Build history of the part. All positions in model axes, mm. Round coordinates to 2 decimals unless told otherwise and drop trailing zeros. Loops run counter-clockwise (first coordinate to the right, second up) from the corner with the lowest first, then second, coordinate; pieces in that order, holes last. Notation, with made-up numbers: (20.25, 50.25) - (52.25, 50.25) arc R7 cw to (52.25, 55.25) - close; hole circle Ø7 at (23, 40.5). An arc over 180 degrees is marked (long way). Use one line per item in the form item = value. Start each with the question number.
Q1. Drill centre lines: line 1 (X direction, y = 1.95, z = -15); line 2 (Z direction, x = 1.5, y = 0.5); line 3 (X direction, y = 2.05, z = 0). Where is each one in solid material? Low to high.
Q2. Pin check, flat tip, straight feed: pin 1 (5 mm diameter, centred on x = 0, z = 30, fed in from +Y). Stop position of the tip, or through.
Q3. Saw through at C-C (x = 26). Give the cut face in (y, z), then the cut area to 3 significant figures.
Q4. Saw through at A-A (y = 1). Give the cut face in (x, z), then the cut area to 3 significant figures.
Q5. Saw through at D-D (z = -15). Give the cut face in (x, y), then the cut area to 3 significant figures.
Q6. Saw through at B-B (z = 30). Give the cut face in (x, y), then the cut area to 3 significant figures.
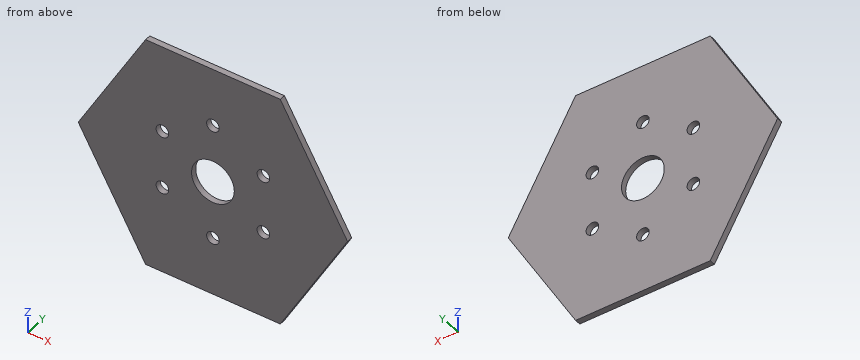
```python
from build123d import *

# Parameters (mm, degrees)
CROQUIS1_R              = 11
SALIENTE_EXTRUIR1_DEPTH = 3
CROQUIS2_R              = 3.25
CORTAR_EXTRUIR1_DEPTH   = 4


with BuildPart() as part:
    # Croquis1 → Saliente-Extruir1 (new body)
    with BuildSketch(Plane(origin=(0, 0, 0), x_dir=(1, 0, 0), z_dir=(0, 1, 0))):
        Polygon((69.282032303, 0), (34.641016151, 60), (-34.641016151, 60), (-69.282032303, 0), (-34.641016151, -60), (34.641016151, -60), align=None)
        Circle(CROQUIS1_R, mode=Mode.SUBTRACT)
    extrude(amount=SALIENTE_EXTRUIR1_DEPTH)

    # Croquis2 → Cortar-Extruir1 (cut, through all)
    with BuildSketch(Plane(origin=(0, 3, 0), x_dir=(1, 0, 0), z_dir=(0, 1, 0))):
        with Locations((0, 30)):
            Circle(CROQUIS2_R)
        with Locations((25.980762114, 15)):
            Circle(CROQUIS2_R)
        with Locations((25.980762114, -15)):
            Circle(CROQUIS2_R)
        with Locations((0, -30)):
            Circle(CROQUIS2_R)
        with Locations((-25.980762114, -15)):
            Circle(CROQUIS2_R)
        with Locations((-25.980762114, 15)):
            Circle(CROQUIS2_R)
    extrude(amount=-CORTAR_EXTRUIR1_DEPTH, mode=Mode.SUBTRACT)


solid = part.part
```
Report:
q1.line_1 = -60.62 to -29.23, -22.73 to 22.73, 29.23 to 60.62
q1.line_2 = -60 to -32.88, -27.12 to -10.9, 10.9 to 27.12, 32.88 to 60
q1.line_3 = -69.28 to -11, 11 to 69.28
q2.pin_1 = through
q3.outline = (0, -60) - (3, -60) - (3, -18.25) - (0, -18.25) - close; (0, -11.75) - (3, -11.75) - (3, 11.75) - (0, 11.75) - close; (0, 18.25) - (3, 18.25) - (3, 60) - (0, 60) - close
q3.area = 321 mm²
q4.outline = (-69.28, 0) - (-34.64, -60) - (34.64, -60) - (69.28, 0) - (34.64, 60) - (-34.64, 60) - close; hole circle Ø6.5 at (-25.98, -15); hole circle Ø6.5 at (-25.98, 15); hole circle Ø22 at (0, 0); hole circle Ø6.5 at (0, -30); hole circle Ø6.5 at (0, 30); hole circle Ø6.5 at (25.98, -15); hole circle Ø6.5 at (25.98, 15)
q4.area = 11,900 mm²
q5.outline = (-60.62, 0) - (-29.23, 0) - (-29.23, 3) - (-60.62, 3) - close; (-22.73, 0) - (22.73, 0) - (22.73, 3) - (-22.73, 3) - close; (29.23, 0) - (60.62, 0) - (60.62, 3) - (29.23, 3) - close
q5.area = 325 mm²
q6.outline = (-51.96, 0) - (-3.25, 0) - (-3.25, 3) - (-51.96, 3) - close; (3.25, 0) - (51.96, 0) - (51.96, 3) - (3.25, 3) - close
q6.area = 292 mm²
